Autodesk Inventor part; units mm, degrees
ref_plane "YZ Plane" through (0, 0, 0) normal (1, 0, 0) x (0, 1, 0)
ref_plane "XZ Plane" through (0, 0, 0) normal (0, 1, 0) x (-1, 0, 0)
ref_plane "XY Plane" through (0, 0, 0) normal (0, 0, 1) x (1, 0, 0)
ref_plane "Work Plane1" through (-35.1299, -83.394, 0) normal (0, 0, 1) x (0.7062905, -0.7079221, 0)
sketch "Sketch1" plane through (-35.1299, -83.394, 0) normal (0, 0, 1) x (0.7062905, -0.7079221, 0)
  circle A0 centre (-118.0078, -0.3279) radius 6.35
  circle A1 centre (-118.5314, 0) radius 149.2286
  arc A2 (48.5793, -75.4462) -> (-285.6421, -75.4462) centre (-118.5314, 0) ccw
  line L0 (-118.5314, 0) -> (-118.5314, 1222.8979) construction
  arc A3 (-244.8846, 1019.4057) -> (7.8218, 1019.4057) centre (-118.5314, 1104.615) ccw
  spline S0 degree 4 poles (7.8218, 1019.4057) (-6.9781, 997.4595) (-39.0532, 578.2178) (-64.4023, 532.3679) (128.916, -51.9504) (48.5793, -75.4462) knots 0 0 0 0 0 0.373535 1 1 1 1 1
  line L1 (25.7608, 1046.0066) -> (-10.1171, 992.8047) construction
  arc A4 (19.6566, 1024.5678) -> (7.4714, 1006.4989) centre (17.8001, 1012.6766) ccw construction
  spline S1 degree 4 poles (-244.8846, 1019.4057) (-230.0846, 997.4595) (-198.0095, 578.2178) (-172.6604, 532.3679) (-365.9787, -51.9504) (-285.6421, -75.4462) knots 0 0 0 0 0 0.373535 1 1 1 1 1
  line L2 (-262.8235, 1046.0066) -> (-226.9456, 992.8047) construction
  arc A5 (-244.5341, 1006.4989) -> (-256.7193, 1024.5678) centre (-254.8628, 1012.6766) ccw construction
  arc A6 (-285.6421, -75.4462) -> (48.5793, -75.4462) centre (-118.5314, 0) ccw
  arc A7 (7.8218, 1019.4057) -> (-244.8846, 1019.4057) centre (-118.5314, 1104.615) ccw
  point P0 (-34.2245, 83.7696)
  point P1 (-21.2914, 810.23)
  point P2 (-21.2914, 520.0523)
  point P3 (59.9573, 110.7433)
  point P4 (-215.7713, 810.23)
  point P5 (-215.7713, 520.0523)
  point P6 (-297.02, 110.7433)
  dimension "d0" = 304.8
extrude "Extrusion1" add sketch "Sketch1" against normal blind 76.2 contours A6 A2 | A2 S1 A3 S0 | A3 A7
properties material "Wood (Cherry)"
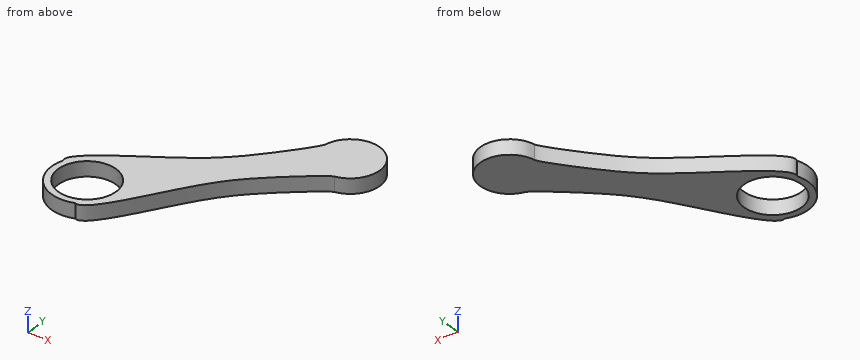
Model file for the job. Use its own axes, mm. Coordinates: 2 decimals unless noted, no trailing zeros. Order: outer loops, then holes, each group sorted by start corner. A loop starts at its lowest first (then second) coordinate and runs counter-clockwise, first axis right, second up. Notation, with made-up numbers: (12, 68.25) -> (42, 68.25) arc R25 ccw to (42, 85.25) -> close; hole circle Ø9 at (76.5, 78). An arc over 180 degrees is marked (long way). Return JSON: item names as keys, results as strings. Group by question number.
Item 1: Flat gauge pins, fed straight in: P1, Ø1.5, axis at x = 142, z = -36.5, coming from the +Y side; P2, Ø1, axis at y = 260.5, z = -40.5, coming from the -X side; P3, Ø6, axis at x = 477.5, z = -12.5, coming from the -Y side; P4, Ø8, axis at x = 562, y = 757.5, coming from the +Z side. Where does each tip first touch, or does it go through?
Item 2: Wall check: line 1 along X through (y, z) = (71.5, -24); line 2 along Y through (x, z) = (-186, -47); line 3 along X through (y, z) = (-110.5, -12.5). Give the ranges that are in metal, low to high. Write a range as [from, to].
Item 3: Saw through at B-B on x = 708.5. Write the cut outline in (y, z), then the cut area to 3 significant figures.
Item 4: Saw through at A-A on y = 854.5. Write the cut outline in (x, z), then the cut area to 3 significant figures.
Values found:
{
 "1": {"P1": "stops at y = 408.29", "P2": "stops at x = -83.62", "P3": "stops at y = 461.54", "P4": "stops at z = 0"},
 "2": {"line 1": "x = [-292.56, -250.11], [12.42, 164.01]", "line 2": "y = [-170.1, -132.75], [133.78, 191.35]", "line 3": "x = [-264.77, -218.57], [-19.13, 38.64]"},
 "3": {"outline": "(635.2, -76.2) -> (926.19, -76.2) -> (926.19, 0) -> (635.2, 0) -> close", "area": "22,200 mm2"},
 "4": {"outline": "(529.8, -76.2) -> (796.47, -76.2) -> (796.47, 0) -> (529.8, 0) -> close", "area": "20,300 mm2"}
}
